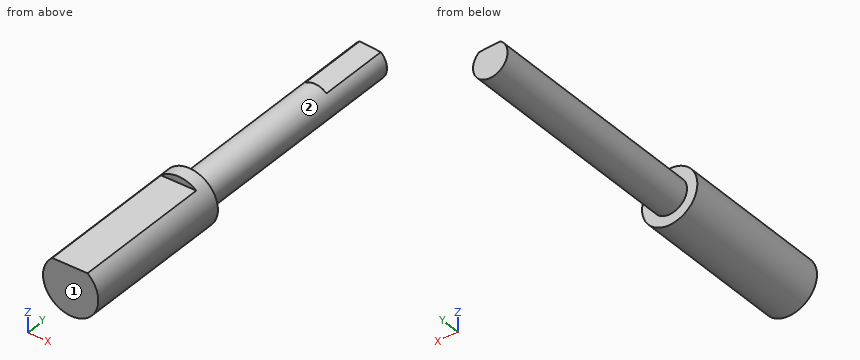
from build123d import *

# Parameters (mm, degrees)
SKETCH1_R           = 4
BOSS_EXTRUDE1_DEPTH = 55
CUT_EXTRUDE1_DEPTH  = 20
CUT_EXTRUDE2_START  = -33
SKETCH3_R           = 4
SKETCH3_R_2         = 2.5
CUT_EXTRUDE2_DEPTH  = 33
CUT_EXTRUDE3_START  = -10
CUT_EXTRUDE3_DEPTH  = 10


with BuildPart() as part:
    # Sketch1 → Boss-Extrude1 (new body)
    with BuildSketch(Plane(origin=(0, 0, 0), x_dir=(1, 0, 0), z_dir=(0, 1, 0))):
        with Locations(Location((0, 0, 0), (0, 0, 270))):
            Circle(SKETCH1_R)
    extrude(amount=BOSS_EXTRUDE1_DEPTH)

    # Sketch2 → Cut-Extrude1 (cut)
    with BuildSketch(Plane.XZ):
        with BuildLine():
            Line((-2.661339853, 2.986179865), (2.444122866, 3.166427547))
            ThreePointArc((2.444122866, 3.166427547), (-0.14113154, 3.997509461), (-2.661339853, 2.986179865))
        make_face()
    extrude(amount=-CUT_EXTRUDE1_DEPTH, mode=Mode.SUBTRACT)

    # Sketch3 → Cut-Extrude2 (cut)
    with BuildSketch(Plane(origin=(0, 55, 0), x_dir=(1, 0, 0), z_dir=(0, 1, 0)).offset(CUT_EXTRUDE2_START)):
        with Locations(Location((0, 0, 0), (0, 0, 228.291972002))):
            Circle(SKETCH3_R)
        with Locations(Location((0, 0, 0), (0, 0, 270))):
            Circle(SKETCH3_R_2, mode=Mode.SUBTRACT)
    extrude(amount=CUT_EXTRUDE2_DEPTH, mode=Mode.SUBTRACT)

    # Sketch6 → Cut-Extrude3 (cut)
    with BuildSketch(Plane(origin=(0, 55, 0), x_dir=(1, 0, 0), z_dir=(0, 1, 0)).offset(CUT_EXTRUDE3_START)):
        with BuildLine():
            Line((-1.479257304, -2.015390242), (1.606973788, -1.915107111))
            ThreePointArc((1.606973788, -1.915107111), (0.081191451, -2.498681242), (-1.479257304, -2.015390242))
        make_face()
    extrude(amount=CUT_EXTRUDE3_DEPTH, mode=Mode.SUBTRACT)


solid = part.part
Verification items for the finished model (mm, model axes). Face numbers are marked on the shaded views. A direction names the side the tool comes from. Round coordinates to 2 decimals unless told otherwise and drop trailing zeros. Order: outer loops, then holes, each group sorted by start corner. A loop starts at its lowest first (then second) coordinate and runs counter-clockwise, first axis right, second up. Notation, with made-up numbers: (73.5, 53.5) -> (106.5, 53.5) arc R18 ccw to (106.5, 68.5) -> close; hole circle Ø6 at (60.5, 36.25). An arc over 180 degrees is marked (long way). Put each result on its own line as item: value.
1) Material ranges on line 1 (Y direction, x = 1.5, z = -3.5); line 2 (Y direction, x = -0.75, z = 3.25); line 3 (Z direction, x = 1.75, y = 24.5), recorded low to high.
Final values:
line 1: y = 0 to 22
line 2: y = 20 to 22
line 3: z = -1.79 to 1.79
2) Section check D-D (x = 3.5). Record the cut outline in (y, z).
Final values:
outline: (0, -1.94) -> (22, -1.94) -> (22, 1.94) -> (0, 1.94) -> close
3) Section check A-A (z = 0). Record the cut outline in (x, y).
Final values:
outline: (-4, 0) -> (4, 0) -> (4, 22) -> (2.5, 22) -> (2.5, 55) -> (-2.5, 55) -> (-2.5, 22) -> (-4, 22) -> close
4) Section check B-B (y = 30). Record the cut outline in (x, z).
Final values:
outline: circle Ø5 at (0, 0)
5) Set-up check for the marked faces 1 and 2: record each of +Z, -Z, +X, -X, +Y, -Y from which the full face is reachable in a straight line by a thin tool's end or side.
Final values:
face 1: +Z, -Z, +X, -X, -Y
face 2: +Y
6) Section check C-C (x = 0). Record the cut outline in (y, z), then the cut area to 3 significant figures.
Final values:
outline: (0, -4) -> (22, -4) -> (22, -2.5) -> (55, -2.5) -> (55, 1.97) -> (45, 1.97) -> (45, 2.5) -> (22, 2.5) -> (22, 4) -> (20, 4) -> (20, 3.08) -> (0, 3.08) -> close
area: 317 mm^2
7) Depth check by flat-ended pin: pin 1 (4 mm diameter, centred on y = 44, z = -1.5, fed in from +X); pin 2 (1 mm diameter, centred on y = 38.5, z = -1, fed in from +X); pin 3 (4 mm diameter, centred on x = -1, y = 46.5, fed in from -Z). Enter the tip coordinate at first touch or a pass-through.
Final values:
pin 1: stops at x = 2.5
pin 2: stops at x = 2.45
pin 3: stops at z = -2.5
